Geometry check sheet. Reference: the model listing, model coordinates, mm. Coordinates: 2 decimals unless noted, no trailing zeros. Write each loop counter-clockwise with the first axis right and the second up, starting at its lowest first coordinate (ties: lowest second). Pieces come first, ordered by that corner, then holes. Notation, with made-up numbers: M 0,85.25 L 35,85.25 A25 cw 35,100.25 Z; hole C -21.5,22.25 d10. An arc over 180 degrees is marked long. Write each question's results on one line, items separated by ' | '.
```python
from build123d import *

# Parameters (mm, degrees)
F0_R     = 35
F0_R_2   = 5
F1_DEPTH = 1.25


with BuildPart() as f1:
    # F0 (on Front) → F1 (new body, symmetric)
    with BuildSketch(Plane.XZ):
        Circle(F0_R)
        with BuildLine():
            Line((-3.375181405, -13.6238082225), (-8.0104363206, -27.8896559669))
            ThreePointArc((-8.0104363206, -27.8896559669), (-9.2705098312, -28.5316954889), (-9.9125493532, -27.2716219782))
            Line((-9.9125493532, -27.2716219782), (-5.2772944375, -13.0057742338))
            ThreePointArc((-5.2772944375, -13.0057742338), (-4.0172209269, -12.3637347118), (-3.375181405, -13.6238082225))
        make_face(mode=Mode.SUBTRACT)
        with BuildLine():
            Line((-13.0057742338, -5.2772944375), (-27.2716219782, -9.9125493532))
            ThreePointArc((-27.2716219782, -9.9125493532), (-28.5316954889, -9.2705098312), (-27.8896559669, -8.0104363206))
            Line((-27.8896559669, -8.0104363206), (-13.6238082225, -3.375181405))
            ThreePointArc((-13.6238082225, -3.375181405), (-12.3637347118, -4.0172209269), (-13.0057742338, -5.2772944375))
        make_face(mode=Mode.SUBTRACT)
        with BuildLine():
            Line((-7.4199765377, -11.9140231735), (-16.2367553221, -24.0492780892))
            ThreePointArc((-16.2367553221, -24.0492780892), (-17.6335575688, -24.2705098312), (-17.8547893109, -22.8737075846))
            Line((-17.8547893109, -22.8737075846), (-9.0380105265, -10.738452669))
            ThreePointArc((-9.0380105265, -10.738452669), (-7.6412082798, -10.5172209269), (-7.4199765377, -11.9140231735))
        make_face(mode=Mode.SUBTRACT)
        with BuildLine():
            Line((-10.738452669, -9.0380105265), (-22.8737075846, -17.8547893109))
            ThreePointArc((-22.8737075846, -17.8547893109), (-24.2705098312, -17.6335575688), (-24.0492780892, -16.2367553221))
            Line((-24.0492780892, -16.2367553221), (-11.9140231735, -7.4199765377))
            ThreePointArc((-11.9140231735, -7.4199765377), (-10.5172209269, -7.6412082798), (-10.738452669, -9.0380105265))
        make_face(mode=Mode.SUBTRACT)
        with BuildLine():
            Line((1, -14), (1, -29))
            ThreePointArc((1, -29), (0, -30), (-1, -29))
            Line((-1, -29), (-1, -14))
            ThreePointArc((-1, -14), (0, -13), (1, -14))
        make_face(mode=Mode.SUBTRACT)
        with BuildLine():
            Line((5.2772944375, -13.0057742338), (9.9125493532, -27.2716219782))
            ThreePointArc((9.9125493532, -27.2716219782), (9.2705098312, -28.5316954889), (8.0104363206, -27.8896559669))
            Line((8.0104363206, -27.8896559669), (3.375181405, -13.6238082225))
            ThreePointArc((3.375181405, -13.6238082225), (4.0172209269, -12.3637347118), (5.2772944375, -13.0057742338))
        make_face(mode=Mode.SUBTRACT)
        with BuildLine():
            Line((9.0380105265, -10.738452669), (17.8547893109, -22.8737075846))
            ThreePointArc((17.8547893109, -22.8737075846), (17.6335575688, -24.2705098312), (16.2367553221, -24.0492780892))
            Line((16.2367553221, -24.0492780892), (7.4199765377, -11.9140231735))
            ThreePointArc((7.4199765377, -11.9140231735), (7.6412082798, -10.5172209269), (9.0380105265, -10.738452669))
        make_face(mode=Mode.SUBTRACT)
        with BuildLine():
            Line((11.9140231735, -7.4199765377), (24.0492780892, -16.2367553221))
            ThreePointArc((24.0492780892, -16.2367553221), (24.2705098312, -17.6335575688), (22.8737075846, -17.8547893109))
            Line((22.8737075846, -17.8547893109), (10.738452669, -9.0380105265))
            ThreePointArc((10.738452669, -9.0380105265), (10.5172209269, -7.6412082798), (11.9140231735, -7.4199765377))
        make_face(mode=Mode.SUBTRACT)
        with BuildLine():
            Line((13.6238082225, -3.375181405), (27.8896559669, -8.0104363206))
            ThreePointArc((27.8896559669, -8.0104363206), (28.5316954889, -9.2705098312), (27.2716219782, -9.9125493532))
            Line((27.2716219782, -9.9125493532), (13.0057742338, -5.2772944375))
            ThreePointArc((13.0057742338, -5.2772944375), (12.3637347118, -4.0172209269), (13.6238082225, -3.375181405))
        make_face(mode=Mode.SUBTRACT)
        with BuildLine():
            Line((-14, -1), (-29, -1))
            ThreePointArc((-29, -1), (-30, 0), (-29, 1))
            Line((-29, 1), (-14, 1))
            ThreePointArc((-14, 1), (-13, 0), (-14, -1))
        make_face(mode=Mode.SUBTRACT)
        with BuildLine():
            Line((-13.6238082225, 3.375181405), (-27.8896559669, 8.0104363206))
            ThreePointArc((-27.8896559669, 8.0104363206), (-28.5316954889, 9.2705098312), (-27.2716219782, 9.9125493532))
            Line((-27.2716219782, 9.9125493532), (-13.0057742338, 5.2772944375))
            ThreePointArc((-13.0057742338, 5.2772944375), (-12.3637347118, 4.0172209269), (-13.6238082225, 3.375181405))
        make_face(mode=Mode.SUBTRACT)
        with BuildLine():
            Line((-11.9140231735, 7.4199765377), (-24.0492780892, 16.2367553221))
            ThreePointArc((-24.0492780892, 16.2367553221), (-24.2705098312, 17.6335575688), (-22.8737075846, 17.8547893109))
            Line((-22.8737075846, 17.8547893109), (-10.738452669, 9.0380105265))
            ThreePointArc((-10.738452669, 9.0380105265), (-10.5172209269, 7.6412082798), (-11.9140231735, 7.4199765377))
        make_face(mode=Mode.SUBTRACT)
        with BuildLine():
            Line((-9.0380105265, 10.738452669), (-17.8547893109, 22.8737075846))
            ThreePointArc((-17.8547893109, 22.8737075846), (-17.6335575688, 24.2705098312), (-16.2367553221, 24.0492780892))
            Line((-16.2367553221, 24.0492780892), (-7.4199765377, 11.9140231735))
            ThreePointArc((-7.4199765377, 11.9140231735), (-7.6412082798, 10.5172209269), (-9.0380105265, 10.738452669))
        make_face(mode=Mode.SUBTRACT)
        with BuildLine():
            Line((-5.2772944375, 13.0057742338), (-9.9125493532, 27.2716219782))
            ThreePointArc((-9.9125493532, 27.2716219782), (-9.2705098312, 28.5316954889), (-8.0104363206, 27.8896559669))
            Line((-8.0104363206, 27.8896559669), (-3.375181405, 13.6238082225))
            ThreePointArc((-3.375181405, 13.6238082225), (-4.0172209269, 12.3637347118), (-5.2772944375, 13.0057742338))
        make_face(mode=Mode.SUBTRACT)
        Circle(F0_R_2, mode=Mode.SUBTRACT)
        with BuildLine():
            Line((10.738452669, 9.0380105265), (22.8737075846, 17.8547893109))
            ThreePointArc((22.8737075846, 17.8547893109), (24.2705098312, 17.6335575688), (24.0492780892, 16.2367553221))
            Line((24.0492780892, 16.2367553221), (11.9140231735, 7.4199765377))
            ThreePointArc((11.9140231735, 7.4199765377), (10.5172209269, 7.6412082798), (10.738452669, 9.0380105265))
        make_face(mode=Mode.SUBTRACT)
        with BuildLine():
            Line((7.4199765377, 11.9140231735), (16.2367553221, 24.0492780892))
            ThreePointArc((16.2367553221, 24.0492780892), (17.6335575688, 24.2705098312), (17.8547893109, 22.8737075846))
            Line((17.8547893109, 22.8737075846), (9.0380105265, 10.738452669))
            ThreePointArc((9.0380105265, 10.738452669), (7.6412082798, 10.5172209269), (7.4199765377, 11.9140231735))
        make_face(mode=Mode.SUBTRACT)
        with BuildLine():
            Line((14, 1), (29, 1))
            ThreePointArc((29, 1), (30, 0), (29, -1))
            Line((29, -1), (14, -1))
            ThreePointArc((14, -1), (13, 0), (14, 1))
        make_face(mode=Mode.SUBTRACT)
        with BuildLine():
            Line((13.0057742338, 5.2772944375), (27.2716219782, 9.9125493532))
            ThreePointArc((27.2716219782, 9.9125493532), (28.5316954889, 9.2705098312), (27.8896559669, 8.0104363206))
            Line((27.8896559669, 8.0104363206), (13.6238082225, 3.375181405))
            ThreePointArc((13.6238082225, 3.375181405), (12.3637347118, 4.0172209269), (13.0057742338, 5.2772944375))
        make_face(mode=Mode.SUBTRACT)
        with BuildLine():
            Line((-1, 14), (-1, 29))
            ThreePointArc((-1, 29), (0, 30), (1, 29))
            Line((1, 29), (1, 14))
            ThreePointArc((1, 14), (0, 13), (-1, 14))
        make_face(mode=Mode.SUBTRACT)
        with BuildLine():
            Line((3.375181405, 13.6238082225), (8.0104363206, 27.8896559669))
            ThreePointArc((8.0104363206, 27.8896559669), (9.2705098312, 28.5316954889), (9.9125493532, 27.2716219782))
            Line((9.9125493532, 27.2716219782), (5.2772944375, 13.0057742338))
            ThreePointArc((5.2772944375, 13.0057742338), (4.0172209269, 12.3637347118), (3.375181405, 13.6238082225))
        make_face(mode=Mode.SUBTRACT)
    extrude(amount=F1_DEPTH, both=True)


solid = f1.part
```
Q1. Sectioned sample at A-A on z = -19. Record the cut outline in (x, y), and give its area (3 significant figures).
Geometry check:
outline: M -29.39,-1.25 L -15.04,-1.25 L -15.04,1.25 L -29.39,1.25 Z; M -12.57,-1.25 L -7.22,-1.25 L -7.22,1.25 L -12.57,1.25 Z; M -5.12,-1.25 L -1,-1.25 L -1,1.25 L -5.12,1.25 Z; M 1,-1.25 L 5.12,-1.25 L 5.12,1.25 L 1,1.25 Z; M 7.22,-1.25 L 12.57,-1.25 L 12.57,1.25 L 7.22,1.25 Z; M 15.04,-1.25 L 29.39,-1.25 L 29.39,1.25 L 15.04,1.25 Z | area: 119 mm2
Q2. Sectioned sample at C-C on y = 0. Give the number of separate pieces and of enclosed holes in the cut face, and give its area (3 significant figures).
Geometry check:
separate pieces: 1 | enclosed holes: 21 | area: 3,110 mm2
Q3. Scan lines: probe 1 along Z at (x, y) = (0, 0.2); probe 2 along Z at (x, y) = (21.5, -1); probe 3 along X at (y, z) = (0.25, 10). Record each from-to range of solid material in increasing order.
Geometry check:
probe 1: z = -35 to -30, -13 to -5, 5 to 13, 30 to 35 | probe 2: z = -27.62 to -16.86, -14.38 to -8.04, -5.93 to -1, 1 to 5.93, 8.04 to 14.38, 16.86 to 27.62 | probe 3: x = -33.54 to -15.47, -12.06 to 12.06, 15.47 to 33.54
Q4. Depth check by flat-ended pin: P1, Ø1.2, axis at y = -0.5, z = 18, coming from the +X side; P2, Ø1, axis at x = 20.5, y = 0.5, coming from the -Z side; P3, Ø0.8, axis at y = 0, z = 22, coming from the -X side; P4, Ø1.5, axis at x = -0.5, z = 25.5, coming from the -Y side. Enter the tip coordinate at first touch or a pass-through.
Geometry check:
P1: stops at x = 30.37 | P2: stops at z = -28.72 | P3: stops at x = -27.54 | P4: stops at y = -1.25
Q5. Sectioned sample at B-B on x = -19. Record the cut outline in (y, z), and give its area (3 significant figures).
Geometry check:
outline: M -1.25,-29.39 L 1.25,-29.39 L 1.25,-15.04 L -1.25,-15.04 Z; M -1.25,-12.57 L 1.25,-12.57 L 1.25,-7.22 L -1.25,-7.22 Z; M -1.25,-5.12 L 1.25,-5.12 L 1.25,-1 L -1.25,-1 Z; M -1.25,1 L 1.25,1 L 1.25,5.12 L -1.25,5.12 Z; M -1.25,7.22 L 1.25,7.22 L 1.25,12.57 L -1.25,12.57 Z; M -1.25,15.04 L 1.25,15.04 L 1.25,29.39 L -1.25,29.39 Z | area: 119 mm2
